Input: dimensioned drawing with shaded views. Units: mm. Origin: part minimum x, y, z. A direction names the side the tool comes from. Coordinates: 2 decimals unless noted, no trailing zeros. Write each loop counter-clockwise with the first axis right and the second up, starting at its lowest first coordinate (ties: lowest second). Pieces come first, ordered by that corner, then holes. Notation, with made-up numbers: (-20, 26) -> (-9, 26) arc R6 ccw to (-9, 37) -> close; hole circle Ø10 at (80.25, 69.5). An arc over 180 degrees is marked (long way). One line per item, written item: value. Start each with the question number.
1. Access query for the marked faces 1, 2, 3, 4 and 5. Directions: +Z, -Z, +X, -X, +Y, -Y. A direction counts if a zero-diameter tool reaches every point of the face in a straight line with its end or side. Return the directions, or none.
2. Section query C-C, the plane x = 76. Output: boundary loops of the cut face in (y, z).
3. First-contact query: P1, Ø3, axis at y = 4, z = 44.5, coming from the +X side; P2, Ø1, axis at y = 2, z = 63.5, coming from the +X side; P3, Ø3, axis at x = 20.5, y = 2, coming from the +Z side. Flat tips, straight axial feed; report the tip coordinate or a pass-through.
4. Section query D-D, the plane z = 22.5. Output: boundary loops of the cut face in (x, y).
5. Line query: line 1 (Y direction, x = 70.5, z = 80.5); line 2 (Z direction, x = 44, y = 4.75) (1 decimal); line 3 (Z direction, x = 76.5, y = 5.5) (1 decimal). Output: solid intervals per line, ascending.
6. Section query B-B, the plane z = 35. Output: boundary loops of the cut face in (x, y).
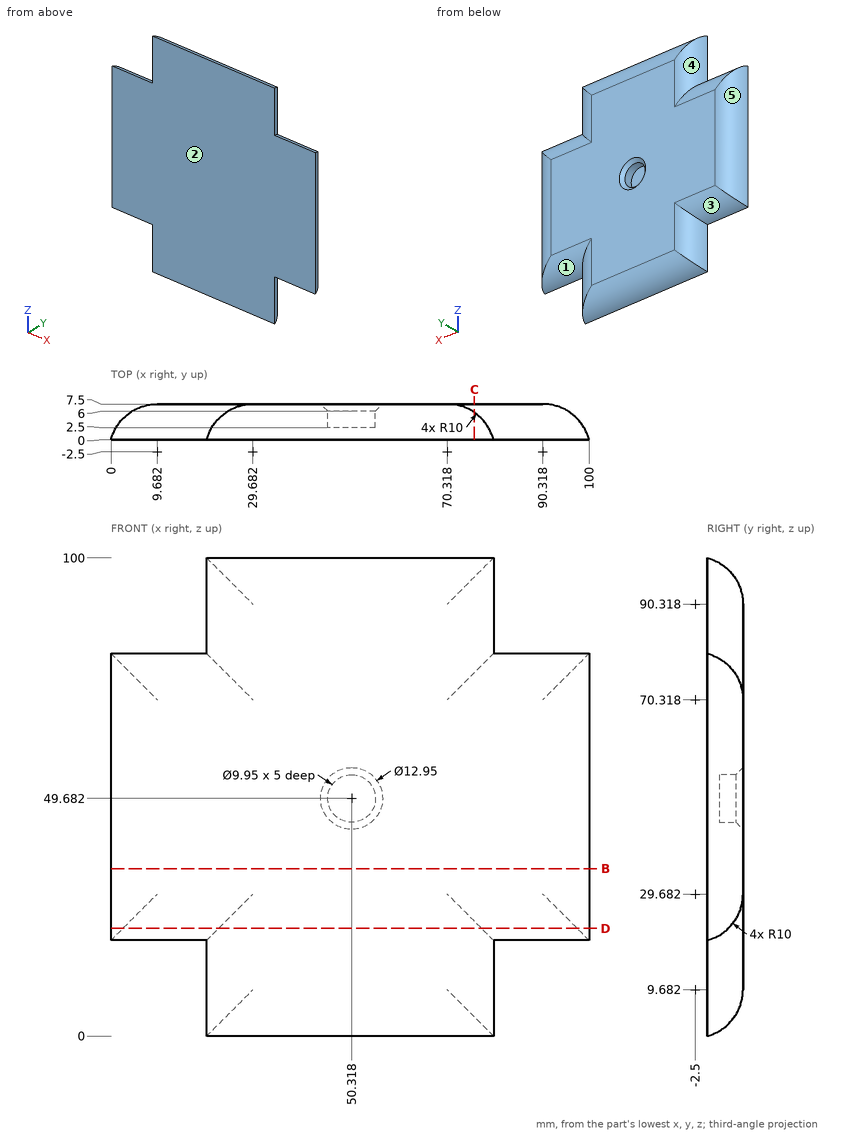
Computed values:
1. face 1: -Z, +X, +Y
1. face 2: +Z, -Z, +X, -X, -Y
1. face 3: -Z, -X, +Y
1. face 4: +Z, -X, +Y
1. face 5: +Z, -Z, -X, +Y
2. outline: (0, 0) arc R10 ccw to (5.73, 4) -> (5.73, 24) arc R10 ccw to (7.5, 29.68) -> (7.5, 70.32) arc R10 ccw to (5.73, 76) -> (5.73, 96) arc R10 ccw to (0, 100) -> close
3. P1: stops at x = 98.98
3. P2: stops at x = 99.48
3. P3: stops at z = 99.86
4. outline: (0, 0) -> (100, 0) arc R10 ccw to (97.5, 4.46) -> (77.5, 4.46) arc R10 ccw to (70.32, 7.5) -> (29.68, 7.5) arc R10 ccw to (22.5, 4.46) -> (2.5, 4.46) arc R10 ccw to start
5. line 1: y = 0 to 7.5
5. line 2: z = 2.8 to 97.2
5. line 3: z = 23.7 to 76.3
6. outline: (0, 0) -> (100, 0) arc R10 ccw to (90.32, 7.5) -> (9.68, 7.5) arc R10 ccw to start
